```python
from build123d import *

# Parameters (mm, degrees)
SKETCH1_W           = 240
SKETCH1_H           = 351.15
BOSS_EXTRUDE3_DEPTH = 21
SKETCH5_W           = 248.975913499
SKETCH5_H           = 113.170869772
CUT_EXTRUDE5_DEPTH  = 254
CAVITY1_START       = -93.176553254
CAVITY1_DEPTH       = 230
SKETCH6_W           = 230
SKETCH6_H           = 2.384694545
CUT_EXTRUDE6_DEPTH  = 10
SKETCH7_W           = 329.692379319
SKETCH7_H           = 158.801284786
CUT_EXTRUDE8_DEPTH  = 33
CUT_EXTRUDE9_DEPTH  = 12
SKETCH15_W          = 230
SKETCH15_H          = 129.5
CUT_EXTRUDE15_DEPTH = 3.5
CUT_EXTRUDE17_DEPTH = 1
CUT_EXTRUDE18_START = -1
CUT_EXTRUDE18_DEPTH = 1
CUT_EXTRUDE19_DEPTH = 1
CUT_EXTRUDE20_START = -1
CUT_EXTRUDE20_DEPTH = 1


with BuildPart() as part:
    # Sketch1 → Boss-Extrude3 (new body)
    with BuildSketch(Plane(origin=(0, 0, 0), x_dir=(1, 0, 0), z_dir=(0, 1, 0))):
        with Locations((21.823446746, 98.176553254)):
            Rectangle(SKETCH1_W, SKETCH1_H)
    extrude(amount=BOSS_EXTRUDE3_DEPTH)

    # Sketch5 → Cut-Extrude5 (cut)
    with BuildSketch(Plane(origin=(0, 0, -54.481553254), x_dir=(-1, 0, 0), z_dir=(0, 0, -1))):
        with Locations((-20.8478358, 4.110963623)):
            Rectangle(SKETCH5_W, SKETCH5_H)
    extrude(amount=CUT_EXTRUDE5_DEPTH, mode=Mode.SUBTRACT)

    # Cavity1: read off the stored shape, not the designer's step
    # Cavity1 outline → Cavity1 (cut)
    with BuildSketch(Plane.YZ.offset(CAVITY1_START)):
        Polygon((18.5, 60.403141291), (13.5, 67.518446746), (13.5, 67.903141291), (18.5, 67.903141291), (13.5, 75.018446746), (5, 75.018446746), (5, -54.481553254), (13.5, -54.481553254), (13.5, -52.096858709), (18.5, -52.096858709), (13.5, -44.981553254), (13.5, -44.596858709), (18.5, -44.596858709), (13.5, -37.481553254), (13.5, -37.096858709), (18.5, -37.096858709), (13.5, -29.981553254), (13.5, -29.596858709), (18.5, -29.596858709), (13.5, -22.481553254), (13.5, -22.096858709), (18.5, -22.096858709), (13.5, -14.981553254), (13.5, -14.596858709), (18.5, -14.596858709), (13.5, -7.481553254), (13.5, -7.096858709), (18.5, -7.096858709), (13.5, 0.018446746), (13.5, 0.403141291), (18.5, 0.403141291), (13.5, 7.518446746), (13.5, 7.903141291), (18.5, 7.903141291), (13.5, 15.018446746), (13.5, 15.403141291), (18.5, 15.403141291), (13.5, 22.518446746), (13.5, 22.903141291), (18.5, 22.903141291), (13.5, 30.018446746), (13.5, 30.403141291), (18.5, 30.403141291), (13.5, 37.518446746), (13.5, 37.903141291), (18.5, 37.903141291), (13.5, 45.018446746), (13.5, 45.403141291), (18.5, 45.403141291), (13.5, 52.518446746), (13.5, 52.903141291), (18.5, 52.903141291), (13.5, 60.018446746), (13.5, 60.403141291), align=None)
    extrude(amount=CAVITY1_DEPTH, mode=Mode.SUBTRACT)

    # Sketch6 → Cut-Extrude6 (cut)
    with BuildSketch(Plane(origin=(0, 13.5, 0), x_dir=(-1, 0, 0), z_dir=(0, -1, 0))):
        with Locations((-21.823446746, 53.289205982)):
            Rectangle(SKETCH6_W, SKETCH6_H)
    extrude(amount=-CUT_EXTRUDE6_DEPTH, mode=Mode.SUBTRACT)

    # Sketch7 → Cut-Extrude8 (cut)
    with BuildSketch(Plane(origin=(0, 13.5, 0), x_dir=(-1, 0, 0), z_dir=(0, -1, 0))):
        with Locations((-33.84938791, -12.885366014)):
            Rectangle(SKETCH7_W, SKETCH7_H)
    extrude(amount=-CUT_EXTRUDE8_DEPTH, mode=Mode.SUBTRACT)

    # Sketch9 → Cut-Extrude9 (cut)
    with BuildSketch(Plane(origin=(0, 13.5, 0), x_dir=(1, 0, 0), z_dir=(0, 1, 0))):
        Polygon((139.223446746, 54.481553254), (139.223446746, -75.718446746), (139.223446746, -77.398446746), (141.823446746, -77.398446746), (141.823446746, 54.481553254), align=None)
        Polygon((-95.576553254, -75.718446746), (-95.576553254, -77.398446746), (-98.176553254, -77.398446746), (-98.176553254, 54.481553254), (-95.576553254, 54.481553254), align=None)
    extrude(amount=-CUT_EXTRUDE9_DEPTH, mode=Mode.SUBTRACT)

    # Sketch15 → Cut-Extrude15 (cut)
    with BuildSketch(Plane(origin=(0, 5, 0), x_dir=(1, 0, 0), z_dir=(0, 1, 0))):
        with Locations((21.823446746, -10.268446746)):
            Rectangle(SKETCH15_W, SKETCH15_H)
    extrude(amount=-CUT_EXTRUDE15_DEPTH, mode=Mode.SUBTRACT)

    # Sketch17 → Cut-Extrude17 (cut)
    with BuildSketch(Plane.ZY.offset(95.576553254)):
        with BuildLine():
            Line((9.418446746, 4.5), (9.526698687, 11.090649814))
            ThreePointArc((9.526698687, 11.090649814), (11.472572716, 13.036523843), (13.418446746, 11.090649814))
            Line((13.418446746, 11.090649814), (13.418446746, 4.5))
            ThreePointArc((13.418446746, 4.5), (11.418446746, 2.5), (9.418446746, 4.5))
        make_face()
    extrude(amount=-CUT_EXTRUDE17_DEPTH, mode=Mode.SUBTRACT)

    # Sketch16 → Cut-Extrude18 (cut)
    with BuildSketch(Plane(origin=(139.223446746, 0, 0), x_dir=(0, 0, -1), z_dir=(1, 0, 0)).offset(CUT_EXTRUDE18_START)):
        with BuildLine():
            Line((-13.418446746, 4.5), (-13.418446746, 11.090649814))
            ThreePointArc((-13.418446746, 11.090649814), (-11.472572716, 13.036523843), (-9.526698687, 11.090649814))
            Line((-9.526698687, 11.090649814), (-9.418446746, 4.5))
            ThreePointArc((-9.418446746, 4.5), (-11.418446746, 2.5), (-13.418446746, 4.5))
        make_face()
    extrude(amount=CUT_EXTRUDE18_DEPTH, mode=Mode.SUBTRACT)

    # Sketch20 → Cut-Extrude19 (cut)
    with BuildSketch(Plane(origin=(139.223446746, 0, 0), x_dir=(0, 0, -1), z_dir=(1, 0, 0))):
        with BuildLine():
            Line((-59.318446746, 4.5), (-59.318446746, 11.09))
            ThreePointArc((-59.318446746, 11.09), (-61.318446746, 13.09), (-63.318446746, 11.09))
            Line((-63.318446746, 11.09), (-63.318446746, 4.5))
            ThreePointArc((-63.318446746, 4.5), (-61.318446746, 2.5), (-59.318446746, 4.5))
        make_face()
    extrude(amount=-CUT_EXTRUDE19_DEPTH, mode=Mode.SUBTRACT)

    # Sketch18 → Cut-Extrude20 (cut)
    with BuildSketch(Plane.ZY.offset(95.576553254).offset(CUT_EXTRUDE20_START)):
        with BuildLine():
            Line((63.318446746, 4.5), (63.318446746, 11.09))
            ThreePointArc((63.318446746, 11.09), (61.318446746, 13.09), (59.318446746, 11.09))
            Line((59.318446746, 11.09), (59.318446746, 4.5))
            ThreePointArc((59.318446746, 4.5), (61.318446746, 2.5), (63.318446746, 4.5))
        make_face()
    extrude(amount=CUT_EXTRUDE20_DEPTH, mode=Mode.SUBTRACT)


solid = part.part
```
Can you work these out from the model? Positions are in its coordinate system, mm. A direction names the side the tool comes from. Give positions to 0.01 mm unless a question says otherwise; leave off trailing zeros. Loops run counter-clockwise (first coordinate to the right, second up) from the corner with the lowest first, then second, coordinate; pieces in that order, holes last. Notation, with made-up numbers: M 3.5,72.5 L 33.5,72.5 A30 cw 33.5,96.5 Z; hole C -39.5,-14.5 d6. An arc over 180 degrees is marked long. Use CSV: the item, a comma, the result in double quotes. Start each with the question number.
1. On a 3-axis mill with a long thin cutter (end or side, diameter ignored), from which of +Z, -Z, +X, -X, +Y, -Y can I reach the whole of each face in a straight line? I mean faces 1 (the face through (20, 8, 75.018)), 2 (the face through (20, 7, 77.398)). Say none if no direction works.
2. If we mould it in two halves opening along X, with no side actions, what happens to faces 3 (the face through (-93.177, 8, 11)), 4 (the face through (-95.577, 2, 12)), 5 (the face through (49, 1, -54.482)), 6 (the face through (139.223, 2, 11))? For each: released by +X, released by -X, zero draft, split by the parting line, or undercut.
3. For P1, Ø6, axis at x = -15, y = 8, coming from the -Z side; P2, Ø2, axis at y = 9.5, z = 11.5, coming from the -X side; P3, Ø5, axis at x = 27.5, z = 47, coming from the +Y side, each with a flat end and sliding along its axis, tell me the tip position at first contact or that it passes through.
4. Imagine slicing it at A-A, the plane x = -63. Write out the boundary of the cut face in (y, z).
5. Imagine slicing it at B-B, the plane z = 28. Write out the boundary of the cut face in (x, y).
6. If I drill on L1, parallel to X at y = 6.25, z = -37; L2, parallel to Y at x = 55, z = -9; L3, parallel to Z at x = 36.5, y = 11, over which ranges is the centre line in solid material (lowest first)?
Response values:
1,face 1,"-Z, +Y"
1,face 2,"+Z, +X, -X, +Y, -Y"
2,face 3,"undercut"
2,face 4,"released by -X"
2,face 5,"zero draft"
2,face 6,"released by +X"
3,P1,"z = 75.02"
3,P2,"x = -94.58"
3,P3,"y = 1.5"
4,outline,"M 0,-54.48 L 1.5,-54.48 L 1.5,75.02 L 13.5,75.02 L 13.5,77.4 L 0,77.4 Z"
5,outline,"M -98.18,0 L 141.82,0 L 141.82,1.5 L 139.22,1.5 L 139.22,13.5 L 136.82,13.5 L 136.82,1.5 L -93.18,1.5 L -93.18,13.5 L -95.58,13.5 L -95.58,1.5 L -98.18,1.5 Z"
6,L1,"-95.58 to -93.18, 136.82 to 139.22"
6,L2,"0 to 1.5"
6,L3,"75.02 to 77.4"
